```python
from build123d import *

# Parameters (mm, degrees)
SFAZOWANIE1_SIZE = 1
SFAZOWANIE2_SIZE = 1


with BuildPart() as part:
    # Szkic1 → Obrót1 (revolve)
    with BuildSketch(Plane(origin=(0, 0, 0), x_dir=(0, 0, -1), z_dir=(1, 0, 0)), mode=Mode.PRIVATE) as obr_t1_sk:
        Polygon((0, 0), (580, 0), (580, 6), (564, 6), (564, 8), (52, 8), (52, 6), (22, 6), (22, 5), (9, 5), (9, 4), (0, 4), align=None)
    revolve(obr_t1_sk.sketch.rotate(Axis((0, 0, 0), (0, 0, -1)), 90), axis=Axis((0, 0, 0), (0, 0, -1)))

    # Sfazowanie1
    sfazowanie1_edges = [part.edges().sort_by_distance(p)[0] for p in [
        (-6, 0, -22),
        (-4, 0, 0),
        (-5, 0, -9),
    ]]
    chamfer(sfazowanie1_edges, length=SFAZOWANIE1_SIZE - 0.0001)  # a hair under: the kernel refuses the full size

    # Sfazowanie2
    sfazowanie2_edges = [part.edges().sort_by_distance(p)[0] for p in [
        (-6, 0, -580),
    ]]
    chamfer(sfazowanie2_edges, length=SFAZOWANIE2_SIZE)


solid = part.part
```
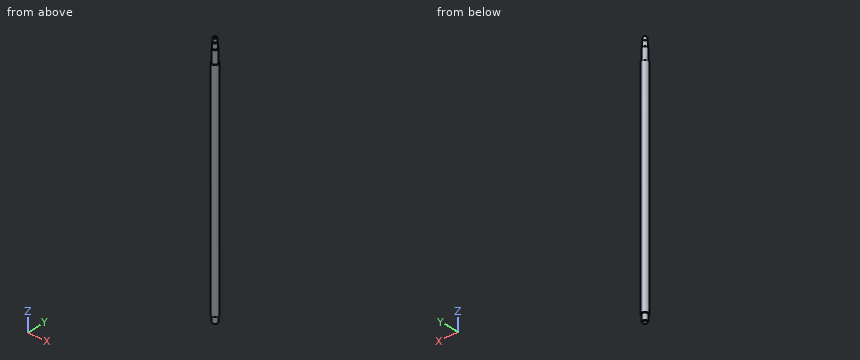
Build history of the part. All positions in model axes, mm. Round coordinates to 2 decimals unless told otherwise and drop trailing zeros. Loops run counter-clockwise (first coordinate to the right, second up) from the corner with the lowest first, then second, coordinate; pieces in that order, holes last.
Item 1: Drill centre lines: line 1 along X through (y, z) = (0.25, -401); line 2 along Y through (x, z) = (-0.75, -31.5); line 3 along Z through (x, y) = (6, -2.75). Where is each one in solid material? Low to high.
Item 2: Saw through at C-C (z = -191.5). List the corners of the cut face in (x, y).
Item 3: Pin check, flat tips, straight feed: P1, Ø3, axis at x = -4, z = -480, coming from the +Y side; P2, Ø1.5, axis at x = -5, z = -135, coming from the -Y side; P3, Ø6.5, axis at x = -0.5, y = -1, coming from the +Z side; P4, Ø4, axis at x = -4, z = -494.5, coming from the +Y side. Stop position of each tip, or through.
Worked answers:
1. line 1: x = -8 to 8
1. line 2: y = -5.95 to 5.95
1. line 3: z = -564 to -52
2. outline: circle Ø16 at (0, 0)
3. P1: stops at y = 7.6
3. P2: stops at y = -6.78
3. P3: stops at z = 0
3. P4: stops at y = 7.75
